from build123d import *

# Parameters (mm, degrees)
SKETCH_1_R          = 7.5
EXTRUDE_1_DEPTH     = 10
SKETCH_5_W          = 30
SKETCH_5_H          = 52
EXTRUDE_2_DEPTH     = 8
SKETCH_6_W          = 30
SKETCH_6_H          = 8
EXTRUDE_3_DEPTH     = 12
SKETCH_7_R          = 55
EXTRUDE_4_DEPTH     = 8
CUT_EXTRUDE_4_REACH = 40
CUT_EXTRUDE_6_DEPTH = 2
CUT_EXTRUDE_7_REACH = 40
SKETCH_12_R         = 9


with BuildPart() as part:
    # 草图1 → 凸台-拉伸1 (new body)
    with BuildSketch(Plane(origin=(0, 0, 0), x_dir=(0, 0, -1), z_dir=(1, 0, 0))):
        Circle(SKETCH_1_R)
    extrude(amount=EXTRUDE_1_DEPTH)

    # 草图5 → 凸台-拉伸2 (add)
    with BuildSketch(Plane(origin=(10, 0, 0), x_dir=(0, 0, -1), z_dir=(1, 0, 0))):
        Rectangle(SKETCH_5_W, SKETCH_5_H)
    extrude(amount=EXTRUDE_2_DEPTH)

    # 草图6 → 凸台-拉伸3 (add)
    with BuildSketch(Plane(origin=(18, 0, 0), x_dir=(0, 0, -1), z_dir=(1, 0, 0))):
        with Locations((0, 22)):
            Rectangle(SKETCH_6_W, SKETCH_6_H)
        with Locations((0, -22)):
            Rectangle(SKETCH_6_W, SKETCH_6_H)
    extrude(amount=EXTRUDE_3_DEPTH)

    # 草图7 → 凸台-拉伸4 (add)
    with BuildSketch(Plane(origin=(30, 0, 0), x_dir=(0, 0, -1), z_dir=(1, 0, 0))):
        Circle(SKETCH_7_R)
    extrude(amount=EXTRUDE_4_DEPTH)

    # 草图8 → 切除-拉伸4 (cut, up to next)
    with BuildSketch(Plane(origin=(38, 0, 0), x_dir=(0, 0, -1), z_dir=(1, 0, 0)), mode=Mode.PRIVATE) as cut_extrude_4_sk1:
        with BuildLine():
            Line((0, 5), (48, 5))
            ThreePointArc((48, 5), (53, 0), (48, -5))
            Line((48, -5), (0, -5))
            ThreePointArc((0, -5), (-5, 0), (0, 5))
        make_face()
    cut_extrude_4_tool1 = extrude(cut_extrude_4_sk1.sketch, amount=-CUT_EXTRUDE_4_REACH, mode=Mode.PRIVATE) & part.part
    add(cut_extrude_4_tool1.solids().sort_by_distance((38, 0, -24))[0], mode=Mode.SUBTRACT)

    # 草图11 → 切除-拉伸6 (cut)
    with BuildSketch(Plane(origin=(38, 0, 0), x_dir=(0, 0, -1), z_dir=(1, 0, 0))):
        with BuildLine():
            Line((0, 7), (54.552726788, 7))
            ThreePointArc((54.552726788, 7), (55, 0), (54.552726788, -7))
            Line((54.552726788, -7), (0, -7))
            ThreePointArc((0, -7), (-7, 0), (0, 7))
        make_face()
    extrude(amount=-CUT_EXTRUDE_6_DEPTH, mode=Mode.SUBTRACT)

    # 草图12 → 切除-拉伸7 (cut, up to next)
    with BuildSketch(Plane.ZY, mode=Mode.PRIVATE) as cut_extrude_7_sk1:
        Circle(SKETCH_12_R)
    cut_extrude_7_tool1 = extrude(cut_extrude_7_sk1.sketch, amount=-CUT_EXTRUDE_7_REACH, mode=Mode.PRIVATE) & part.part
    add(cut_extrude_7_tool1.solids().sort_by_distance((0, 0, 0))[0], mode=Mode.SUBTRACT)


solid = part.part
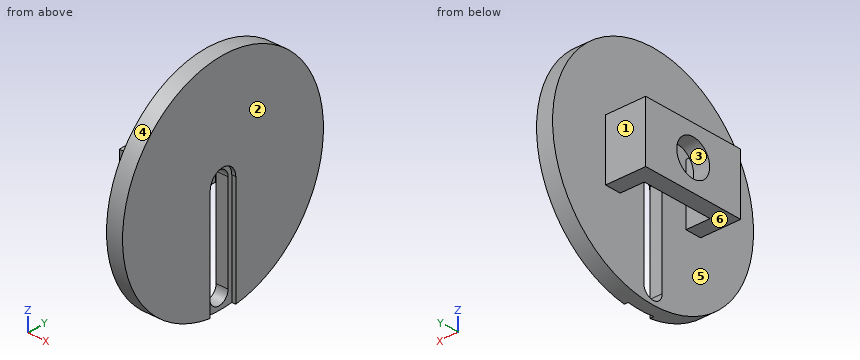
Design review of the part built by this model. Coordinates are the model's own, in mm. Face numbers are marked on the shaded views. A direction names the side the tool comes from. Round coordinates to 2 decimals unless told otherwise and drop trailing zeros. Write each loop counter-clockwise with the first axis right and the second up, starting at its lowest first coordinate (ties: lowest second). Pieces come first, ordered by that corner, then holes. Notation, with made-up numbers: M 25,-32 L 30,-32 A17 cw 30,-5 Z; hole C 43.5,3.25 d7. An arc over 180 degrees is marked long. One line per item, written item: value. Start each with the question number.
1. For the marked faces 1 and 2, list the 3-axis set-ups (+Z, -Z, +X, -X, +Y, -Y) from which the entire face can be reached by the end or side of a thin tool; tool diameter is ignored.
2. Take a section at B-B on y = 0. State the section outline as (x, z) points.
3. Clearance check with flat-ended pins moving along their axes: P1, Ø13, axis at x = 25.5, z = -1.5, coming from the +Y side; P2, Ø4, axis at x = 27.5, y = -13, coming from the -Z side; P3, Ø8, axis at x = 28, z = 25.5, coming from the +Y side; P4, Ø5, axis at x = 32, z = -21, coming from the +Y side. State where each tip first meets the part, or that it passes through.
4. Take a section at A-A on x = 27.5. State the section outline as (y, z) points, then the cut area to 3 significant figures.
5. Take a section at C-C on z = -2. State the section outline as (x, y) points, then the cut area to 3 significant figures.
6. To check wall thickness, follow probe 1 along Y at (x, z) = (12.25, 0); probe 2 along X at (y, z) = (15.5, -5.5); probe 3 along X at (y, z) = (-21, 33). State the ranges of each line that lie inside material, in increasing order. Write a range as from..to.
7. Draft analysis for pull direction Z (two halves, no side actions). For the marked faces 3, 4, 5 and 6, state which applies: pulls with the +Z half, pulls with the -Z half, needs draft (parallel to the pull), parting line crosses it, or undercut.
8. Take a section at D-D on x = 33.25. State the section outline as (y, z) points, then the cut area to 3 significant figures.
Computed:
1. face 1: +Z, -Z, -X, +Y
1. face 2: +Z, -Z, +X, +Y, -Y
2. outline: M 10,-15 L 18,-15 L 18,-9 L 10,-9 Z; M 10,9 L 18,9 L 18,15 L 10,15 Z; M 30,-55 L 36,-55 L 36,-53 L 30,-53 Z; M 30,5 L 36,5 L 36,7 L 38,7 L 38,55 L 30,55 Z
3. P1: stops at y = 55
3. P2: passes through
3. P3: stops at y = 50.39
3. P4: stops at y = 51.8
4. outline: M -26,-15 L -18,-15 L -18,15 L -26,15 Z; M 18,-15 L 26,-15 L 26,15 L 18,15 Z
4. area: 480 mm²
5. outline: M 10,-26 L 30,-26 L 30,-54.96 L 38,-54.96 L 38,-7 L 36,-7 L 36,-5 L 30,-5 L 30,-18 L 18,-18 L 18,-8.77 L 10,-8.77 Z; M 10,8.77 L 18,8.77 L 18,18 L 30,18 L 30,5 L 36,5 L 36,7 L 38,7 L 38,54.96 L 30,54.96 L 30,26 L 10,26 Z
5. area: 1,260 mm²
6. probe 1: y = -26..-9, 9..26
6. probe 2: x = 10..18, 30..38
6. probe 3: x = 30..38
7. face 3: undercut
7. face 4: parting line crosses it
7. face 5: needs draft
7. face 6: pulls with the -Z half
8. outline: C 0,0 d110; hole M -5,-48 A5 ccw 5,-48 L 5,0 A5 ccw -5,0 Z
8. area: 8,940 mm²
